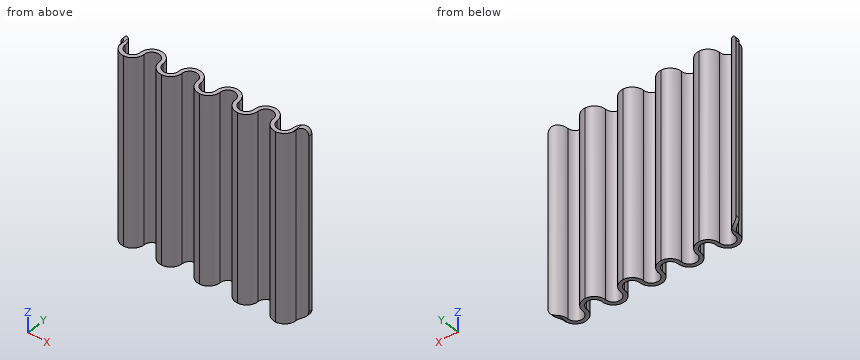
from build123d import *

# Parameters (mm, degrees)
BOSS_EXTRUDE3_DEPTH = 51.43
CUT_EXTRUDE1_DEPTH  = 10


with BuildPart() as part:
    # Sketch2 → Boss-Extrude3 (new body)
    with BuildSketch(Plane.XY):
        with BuildLine():
            ThreePointArc((44.414999988, 3.116666665), (43.502149457, 5.320482799), (41.298333323, 6.23333333))
            ThreePointArc((41.298333323, 6.23333333), (39.09451719, 5.320482799), (38.181666658, 3.116666665))
            ThreePointArc((38.181666658, 3.116666665), (36.103888882, 1.038888889), (34.026111106, 3.116666665))
            ThreePointArc((34.026111106, 3.116666665), (33.113260575, 5.320482799), (30.909444441, 6.23333333))
            ThreePointArc((30.909444441, 6.23333333), (28.705628308, 5.320482799), (27.792777776, 3.116666665))
            ThreePointArc((27.792777776, 3.116666665), (25.715, 1.038888889), (23.637222224, 3.116666665))
            ThreePointArc((23.637222224, 3.116666665), (22.724371692, 5.320482799), (20.520555559, 6.23333333))
            ThreePointArc((20.520555559, 6.23333333), (18.316739425, 5.320482799), (17.403888894, 3.116666665))
            ThreePointArc((17.403888894, 3.116666665), (15.326111118, 1.038888889), (13.248333342, 3.116666665))
            ThreePointArc((13.248333342, 3.116666665), (12.33548281, 5.320482799), (10.131666677, 6.23333333))
            ThreePointArc((10.131666677, 6.23333333), (7.927850543, 5.320482799), (7.015000012, 3.116666665))
            ThreePointArc((7.015000012, 3.116666665), (4.937222236, 1.038888889), (2.859444459, 3.116666665))
            ThreePointArc((2.859444459, 3.116666665), (2.035732981, 5.227582962), (0, 6.222700766))
            Line((0, 6.222700766), (0, 5.178461326))
            ThreePointArc((0, 5.178461326), (1.300277565, 4.491932077), (1.820555571, 3.116666665))
            ThreePointArc((1.820555571, 3.116666665), (2.733406114, 0.91285052), (4.937222268, 0))
            ThreePointArc((4.937222268, 0), (7.141038381, 0.912850543), (8.053888901, 3.116666665))
            ThreePointArc((8.053888901, 3.116666665), (10.131666677, 5.194444441), (12.209444453, 3.116666665))
            ThreePointArc((12.209444453, 3.116666665), (13.122294999, 0.912850517), (15.326111158, 0))
            ThreePointArc((15.326111158, 0), (17.529927266, 0.912850546), (18.442777783, 3.116666665))
            ThreePointArc((18.442777783, 3.116666665), (20.520555559, 5.194444441), (22.598333335, 3.116666665))
            ThreePointArc((22.598333335, 3.116666665), (23.511183872, 0.912850526), (25.715000016, 0))
            ThreePointArc((25.715000016, 0), (27.918816139, 0.912850537), (28.831666665, 3.116666665))
            ThreePointArc((28.831666665, 3.116666665), (30.909444441, 5.194444441), (32.987222217, 3.116666665))
            ThreePointArc((32.987222217, 3.116666665), (33.900072749, 0.912850531), (36.103888882, 0))
            ThreePointArc((36.103888882, 0), (38.307705016, 0.912850531), (39.220555547, 3.116666665))
            ThreePointArc((39.220555547, 3.116666665), (41.298333323, 5.194444441), (43.376111099, 3.116666665))
            ThreePointArc((43.376111099, 3.116666665), (44.288961637, 0.912850526), (46.492777781, 0))
            ThreePointArc((46.492777781, 0), (48.696593904, 0.912850537), (49.609444429, 3.116666665))
            ThreePointArc((49.609444429, 3.116666665), (50.129722435, 4.491932077), (51.43, 5.178461326))
            Line((51.43, 5.178461326), (51.43, 6.222700766))
            ThreePointArc((51.43, 6.222700766), (49.394267019, 5.227582962), (48.570555541, 3.116666665))
            ThreePointArc((48.570555541, 3.116666665), (46.492777764, 1.038888889), (44.414999988, 3.116666665))
        make_face()
    extrude(amount=BOSS_EXTRUDE3_DEPTH)

    # Sketch3 → Cut-Extrude1 (cut)
    with BuildSketch(Plane(origin=(0, 6.23333333, 0), x_dir=(1, 0, 0), z_dir=(0, 1, 0))):
        with BuildLine():
            Line((51.43, -49.43), (51.43, -51.43))
            Line((51.43, -51.43), (49.43, -51.43))
            ThreePointArc((49.43, -51.43), (50.844213562, -50.844213562), (51.43, -49.43))
        make_face()
        with BuildLine():
            Line((51.43, 0), (49.43, 0))
            ThreePointArc((49.43, 0), (50.844213562, -0.585786438), (51.43, -2))
            Line((51.43, -2), (51.43, 0))
        make_face()
        with BuildLine():
            Line((0, 0), (0, -2))
            ThreePointArc((0, -2), (0.585786438, -0.585786438), (2, 0))
            Line((2, 0), (0, 0))
        make_face()
        with BuildLine():
            Line((0, -49.43), (0, -51.43))
            Line((0, -51.43), (2, -51.43))
            ThreePointArc((2, -51.43), (0.585786438, -50.844213562), (0, -49.43))
        make_face()
    extrude(amount=-CUT_EXTRUDE1_DEPTH, mode=Mode.SUBTRACT)


solid = part.part
Geometry: final body of the model. Coordinates: model frame, mm. Coordinates: 2 decimals unless noted, no trailing zeros. Order: outer loops, then holes, each group sorted by start corner. A loop starts at its lowest first (then second) coordinate and runs counter-clockwise, first axis right, second up.
1) Ray query, probe 1 along X at (y, z) = (5.25, 30.5); probe 2 along X at (y, z) = (5.75, 14); probe 3 along X at (y, z) = (1, 49). Return the intervals inside material, ascending.
Result sheet:
probe 1: x = 0 to 2.01, 7.86 to 12.4, 18.25 to 22.79, 28.64 to 33.18, 39.03 to 43.57, 49.42 to 51.43
probe 2: x = 0 to 1.41, 8.46 to 11.8, 18.85 to 22.19, 29.24 to 32.58, 39.63 to 42.97, 50.02 to 51.43
probe 3: x = 2.65 to 7.22, 13.04 to 17.61, 23.43 to 28, 33.82 to 38.39, 44.21 to 48.78
2) Section B-B (x = 26.5). Return loops of the section in (y, z), then the cut area to 3 significant figures.
Result sheet:
outline: (0.1, 0) - (1.19, 0) - (1.19, 51.43) - (0.1, 51.43) - close
area: 56.2 mm2
3) First-contact query: P1, Ø4, axis at x = 30.5, z = 15, coming from the -Y side; P2, Ø1.5, axis at x = 35.5, z = 36, coming from the +Y side; P3, Ø8, axis at x = 30, z = 40.5, coming from the -Y side. Flat tips, straight axial feed; report the tip coordinate or a pass-through.
Result sheet:
P1: stops at y = 1.72
P2: stops at y = 1.54
P3: stops at y = 0.01
